```python
from build123d import *

# Parameters (mm, degrees)
SKETCH2_R           = 1.5
BOSS_EXTRUDE1_DEPTH = 3


with BuildPart() as part:
    # Sketch2 → Boss-Extrude1 (new body)
    with BuildSketch(Plane.XY):
        with BuildLine():
            Line((2.936670729, 6.354601878), (23.677794427, 13.984528989))
            ThreePointArc((23.677794427, 13.984528989), (27.248698254, 13.925360384), (29.850364144, 11.47869129))
            ThreePointArc((29.850364144, 11.47869129), (30.588272685, 10.65075377), (31.653840565, 10.343256382))
            Line((31.653840565, 10.343256382), (45.495725577, 10.343256382))
            Line((45.495725577, 10.343256382), (48.695725577, 14.288892686))
            Line((48.695725577, 14.288892686), (48.964283059, 14.288892686))
            Line((48.964283059, 14.288892686), (49.101750655, 14.15142509))
            Line((49.101750655, 14.15142509), (49.250184878, 14.15142509))
            Line((49.250184878, 14.15142509), (49.387652474, 14.288892686))
            Line((49.387652474, 14.288892686), (49.694283059, 14.288892686))
            Line((49.694283059, 14.288892686), (49.831750655, 14.15142509))
            Line((49.831750655, 14.15142509), (49.980184878, 14.15142509))
            Line((49.980184878, 14.15142509), (50.117652474, 14.288892686))
            Line((50.117652474, 14.288892686), (50.424283059, 14.288892686))
            Line((50.424283059, 14.288892686), (50.561750655, 14.15142509))
            Line((50.561750655, 14.15142509), (50.710184878, 14.15142509))
            Line((50.710184878, 14.15142509), (50.847652474, 14.288892686))
            Line((50.847652474, 14.288892686), (51.154283059, 14.288892686))
            Line((51.154283059, 14.288892686), (51.291750655, 14.15142509))
            Line((51.291750655, 14.15142509), (51.440184878, 14.15142509))
            Line((51.440184878, 14.15142509), (51.577652474, 14.288892686))
            Line((51.577652474, 14.288892686), (51.884283059, 14.288892686))
            Line((51.884283059, 14.288892686), (52.021750655, 14.15142509))
            Line((52.021750655, 14.15142509), (52.170184878, 14.15142509))
            Line((52.170184878, 14.15142509), (52.307652474, 14.288892686))
            Line((52.307652474, 14.288892686), (52.614283059, 14.288892686))
            Line((52.614283059, 14.288892686), (52.751750655, 14.15142509))
            Line((52.751750655, 14.15142509), (52.900184878, 14.15142509))
            Line((52.900184878, 14.15142509), (53.037652474, 14.288892686))
            Line((53.037652474, 14.288892686), (53.344283059, 14.288892686))
            Line((53.344283059, 14.288892686), (53.481750655, 14.15142509))
            Line((53.481750655, 14.15142509), (53.630184878, 14.15142509))
            Line((53.630184878, 14.15142509), (53.767652474, 14.288892686))
            Line((53.767652474, 14.288892686), (54.074283059, 14.288892686))
            Line((54.074283059, 14.288892686), (54.211750655, 14.15142509))
            Line((54.211750655, 14.15142509), (54.360184878, 14.15142509))
            Line((54.360184878, 14.15142509), (54.497652474, 14.288892686))
            Line((54.497652474, 14.288892686), (54.804283059, 14.288892686))
            Line((54.804283059, 14.288892686), (54.941750655, 14.15142509))
            Line((54.941750655, 14.15142509), (55.090184878, 14.15142509))
            Line((55.090184878, 14.15142509), (55.227652474, 14.288892686))
            Line((55.227652474, 14.288892686), (55.534283059, 14.288892686))
            Line((55.534283059, 14.288892686), (55.671750655, 14.15142509))
            Line((55.671750655, 14.15142509), (55.820184878, 14.15142509))
            Line((55.820184878, 14.15142509), (55.957652474, 14.288892686))
            Line((55.957652474, 14.288892686), (56.264283059, 14.288892686))
            Line((56.264283059, 14.288892686), (56.401750655, 14.15142509))
            Line((56.401750655, 14.15142509), (56.550184878, 14.15142509))
            Line((56.550184878, 14.15142509), (56.687652474, 14.288892686))
            Line((56.687652474, 14.288892686), (56.994283059, 14.288892686))
            Line((56.994283059, 14.288892686), (57.131750655, 14.15142509))
            Line((57.131750655, 14.15142509), (57.280184878, 14.15142509))
            Line((57.280184878, 14.15142509), (57.417652474, 14.288892686))
            Line((57.417652474, 14.288892686), (57.724283059, 14.288892686))
            Line((57.724283059, 14.288892686), (57.861750655, 14.15142509))
            Line((57.861750655, 14.15142509), (58.010184878, 14.15142509))
            Line((58.010184878, 14.15142509), (58.147652474, 14.288892686))
            Line((58.147652474, 14.288892686), (58.454283059, 14.288892686))
            Line((58.454283059, 14.288892686), (58.591750655, 14.15142509))
            Line((58.591750655, 14.15142509), (58.740184878, 14.15142509))
            Line((58.740184878, 14.15142509), (58.877652474, 14.288892686))
            Line((58.877652474, 14.288892686), (59.095725577, 14.288892686))
            Line((59.095725577, 14.288892686), (59.095725577, 13.193256382))
            ThreePointArc((59.095725577, 13.193256382), (56.606133217, 7.182848742), (50.595725577, 4.693256382))
            Line((50.595725577, 4.693256382), (28.876707599, 4.693256382))
            ThreePointArc((28.876707599, 4.693256382), (27.123316378, 4.538337348), (25.424251892, 4.078380228))
            Line((25.424251892, 4.078380228), (6.354601878, -2.936670729))
            ThreePointArc((6.354601878, -2.936670729), (0, 0), (2.936670729, 6.354601878))
        make_face()
        with Locations((4.645636304, 1.708965575)):
            Circle(SKETCH2_R, mode=Mode.SUBTRACT)
        with Locations((25.386760002, 9.338892686)):
            Circle(SKETCH2_R, mode=Mode.SUBTRACT)
        with Locations((52.307652474, 9.994763619)):
            Circle(SKETCH2_R, mode=Mode.SUBTRACT)
    extrude(amount=BOSS_EXTRUDE1_DEPTH)


solid = part.part
```
CAD build for the part. Positions are in the model's coordinates, mm. A direction names the side the tool comes from. Round coordinates to 2 decimals unless told otherwise and drop trailing zeros. Order: outer loops, then holes, each group sorted by start corner. A loop starts at its lowest first (then second) coordinate and runs counter-clockwise, first axis right, second up. Notation, with made-up numbers: (3.5, 14) -> (44.5, 14) arc R23 ccw to (44.5, 51) -> close; hole circle Ø10 at (8.25, -15). An arc over 180 degrees is marked (long way). Write item = value, one per line.
(1) Cut at B-B (x = 5.5). Write the cut outline in (y, z), plus the area to 3 significant figures.
Answers follow:
outline = (-3.17, 0) -> (0.48, 0) -> (0.48, 3) -> (-3.17, 3) -> close; (2.94, 0) -> (7.3, 0) -> (7.3, 3) -> (2.94, 3) -> close
area = 24.0 mm²
(2) 3-axis set-ups, long thin cutter, end or side, ignore diameter. For faces 1 (the flat face through (30, 8, 0)), 2 (the flat face through (40, 4.693, 1)), 3 (the cylindrical face through (30.575, 10.659, 1.479)): which of +Z, -Z, +X, -X, +Y, -Y reach the whole face in a straight line?
Answers follow:
face_1 = -Z, +X, -X, +Y, -Y
face_2 = +Z, -Z, +X, -Y
face_3 = +Z, -Z, +Y
(3) Pull direction X, two halves, no side cores. Call faces 4 (the flat face through (30, 8, 3)), 5 (the cylindrical face through (26.817, 9.789, 1.479)), 6 (the flat face through (16.02, 0.62, 1.48)): +X half, -X half, draft (parallel to the pull), parting line (faces both ways), or undercut.
Answers follow:
face_4 = draft
face_5 = undercut
face_6 = +X half
(4) Cut at A-A (y = 12.5). Write the cut outline in (x, z).
Answers follow:
outline = (19.64, 0) -> (29.2, 0) -> (29.2, 3) -> (19.64, 3) -> close; (47.24, 0) -> (59.07, 0) -> (59.07, 3) -> (47.24, 3) -> close
(5) Cut at C-C (x = 40). Write the cut outline in (y, z), plus the area to 4 significant figures.
Answers follow:
outline = (4.69, 0) -> (10.34, 0) -> (10.34, 3) -> (4.69, 3) -> close
area = 16.95 mm²
(6) Cut at D-D (z = 1.75). State how many separate pieces and enclosed holes the cut face has, plus the area to 3 significant figures.
Answers follow:
separate_pieces = 1
enclosed_holes = 3
area = 473 mm²
(7) Drill centre lines: L1, parallel to Y at x = 36, z = 0.85; L2, parallel to Y at x = 52, z = 1.65; L3, parallel to Y at x = 26, z = 2.45. Where is each one in solid material? Low to high.
Answers follow:
L1 = 4.69 to 10.34
L2 = 4.81 to 8.53, 11.46 to 14.17
L3 = 4.27 to 7.97, 10.71 to 14.25
(8) Flat gauge pins, fed straight in: P1, Ø2.5, axis at x = 52.31, y = 9.99, coming from the -Z side; P2, Ø5, axis at x = 36, y = 11, coming from the +Z side. Where does each tip first touch, or does it go through?
Answers follow:
P1 = through
P2 = 3
